Autodesk Inventor part; units mm, degrees
ref_plane "YZ Plane" through (0, 0, 0) normal (1, 0, 0) x (0, 1, 0)
ref_plane "XZ Plane" through (0, 0, 0) normal (0, 1, 0) x (-1, 0, 0)
ref_plane "XY Plane" through (0, 0, 0) normal (0, 0, 1) x (1, 0, 0)
sketch "スケッチ1" plane through (0, 0, 0) normal (0, 0, 1) x (1, 0, 0)
  line L0 (0, 0) -> (-15, 0)
  line L1 (-15, 0) -> (-15, 20)
  line L2 (-15, 20) -> (0, 20)
  line L3 (0, 20) -> (0, 0)
  line L4 (0, 0) -> (0, 43.6966) construction
  line L5 (-15, 12.5) -> (-20, 12.5)
  line L6 (-20, 12.5) -> (-20, 0)
  line L7 (-30, 0) -> (-30, 12.5)
  line L8 (-30, 0) -> (-20, 0)
  line L9 (23.8812, 0) -> (-169.724, 0) construction
  line L10 (-45, 0) -> (-45, 12.5)
  line L11 (-45, 0) -> (-35, 0)
  line L12 (-35, 12.5) -> (-35, 0)
  line L13 (-30, 12.5) -> (-35, 12.5)
  line L14 (-60, 0) -> (-60, 12.5)
  line L15 (-60, 0) -> (-50, 0)
  line L16 (-50, 12.5) -> (-50, 0)
  line L17 (-45, 12.5) -> (-50, 12.5)
  line L18 (-75, 0) -> (-75, 12.5)
  line L19 (-75, 0) -> (-65, 0)
  line L20 (-65, 12.5) -> (-65, 0)
  line L21 (-60, 12.5) -> (-65, 12.5)
  line L22 (-75, 0) -> (-80, 0)
  line L23 (-80, 0) -> (-80, 20)
  line L24 (-80, 20) -> (-75, 20)
  line L25 (-75, 20) -> (-75, 0)
  line L26 (-75, 20) -> (-15, 20)
  line L27 (-75, 0) -> (-80, 5)
  line L28 (-75, 0) -> (-67.9289, 0) construction
  line L29 (0, 5) -> (-5, 0)
  point P0 (-5, 0)
  dimension "d1" = 15
  dimension "d2" = 20
  dimension "d3" = 5
  dimension "d4" = 10
  dimension "d5" = 7.5
  dimension "d8" = 15
  dimension "d13" = 5
  dimension "d14" = 135
  dimension "d15" = 5
  dimension "d16" = 135
extrude "押し出し1" add sketch "スケッチ1" along normal blind 10 contours L0 L29 L3 | L0 L1 L2 L3 L29 | L5 L6 L8 L7 L13 L12 L11 L10 L17 L16 L15 L14 L21 L20 L19 L18 L25 L26 L1 | L25 L18 L27 L23 L24
sketch "スケッチ2" plane through (0, 0, 0) normal (0, 0, -1) x (-1, 0, 0)
  line L0 (80, 20) -> (80, 5)
  line L1 (0, 20) -> (80, 20)
  line L2 (0, 0) -> (0, 20)
  line L3 (15, 0) -> (0, 0)
  line L4 (15, 12.5) -> (15, 0)
  line L5 (20, 12.5) -> (15, 12.5)
  line L6 (20, 0) -> (20, 12.5)
  line L7 (30, 0) -> (20, 0)
  line L8 (30, 12.5) -> (30, 0)
  line L9 (35, 12.5) -> (30, 12.5)
  line L10 (35, 0) -> (35, 12.5)
  line L11 (45, 0) -> (35, 0)
  line L12 (45, 12.5) -> (45, 0)
  line L13 (50, 12.5) -> (45, 12.5)
  line L14 (50, 0) -> (50, 12.5)
  line L15 (60, 0) -> (50, 0)
  line L16 (60, 12.5) -> (60, 0)
  line L17 (65, 12.5) -> (60, 12.5)
  line L18 (65, 0) -> (65, 12.5)
  line L19 (75, 0) -> (65, 0)
  line L20 (80, 5) -> (75, 0)
  line L21 (40, 31.6917) -> (40, -9.5966) construction
  line L22 (42.5, 5) -> (37.5, 5)
  line L23 (37.5, 5) -> (37.5, 17.5)
  line L24 (37.5, 17.5) -> (42.5, 17.5)
  line L25 (42.5, 17.5) -> (42.5, 5)
  line L26 (42.5, 5) -> (37.5, 17.5) construction
  line L27 (37.5, 5) -> (42.5, 17.5) construction
  line L28 (-3.4293, 0) -> (98.1355, 0) construction
  line L29 (52.5, 5) -> (52.5, 17.5)
  line L30 (57.5, 5) -> (52.5, 5)
  line L31 (57.5, 17.5) -> (57.5, 5)
  line L32 (67.5, 5) -> (67.5, 17.5)
  line L33 (72.5, 5) -> (67.5, 5)
  line L34 (72.5, 17.5) -> (72.5, 5)
  line L35 (22.5, 5) -> (22.5, 17.5)
  line L36 (27.5, 5) -> (22.5, 5)
  line L37 (27.5, 17.5) -> (27.5, 5)
  line L38 (37.5, 5) -> (37.5, 17.5)
  line L39 (42.5, 5) -> (37.5, 5)
  line L40 (42.5, 17.5) -> (42.5, 5)
  line L41 (52.5, 5) -> (52.5, 17.5)
  line L42 (57.5, 5) -> (52.5, 5)
  line L43 (57.5, 17.5) -> (57.5, 5)
  line L44 (7.5, 5) -> (7.5, 17.5)
  line L45 (12.5, 5) -> (7.5, 5)
  line L46 (12.5, 17.5) -> (12.5, 5)
  line L47 (22.5, 5) -> (22.5, 17.5)
  line L48 (27.5, 5) -> (22.5, 5)
  line L49 (27.5, 17.5) -> (27.5, 5)
  line L50 (37.5, 5) -> (37.5, 17.5)
  line L51 (42.5, 5) -> (37.5, 5)
  line L52 (42.5, 17.5) -> (42.5, 5)
  line L53 (72.5, 17.5) -> (7.5, 17.5)
  line L54 (7.5, 15) -> (72.5, 15)
  point P0 (40, 11.25)
  point P1 (12.5, 15)
  point P2 (22.5, 15)
  point P3 (27.5, 15)
  point P4 (37.5, 15)
  point P5 (42.5, 15)
  point P6 (52.5, 15)
  point P7 (57.5, 15)
  point P8 (67.5, 15)
  dimension "d19" = 5
  dimension "d20" = 5
  dimension "d21" = 12.5
  dimension "d22" = 5
  dimension "d25" = 15
  dimension "d28" = 15
  dimension "d31" = 2.5
extrude "押し出し2" cut sketch "スケッチ2" against normal blind 7.5 contours L22 L23 L54 L25 | L54 L23 L24 L25 | L25 L53 L29 L54 | L54 L37 L53 L23 | L54 L31 L30 L29 | L29 L53 L31 L54 | L54 L35 L53 L37 | L37 L36 L35 L54 | L31 L53 L32 L54 | L54 L46 L53 L35 | L54 L34 L33 L32 | L32 L53 L34 L54 | L54 L44 L53 L46 | L46 L45 L44 L54
mirror "ミラー2" about plane through (-40, 10, 0) normal (0, 0, -1) of "押し出し1", "押し出し2"
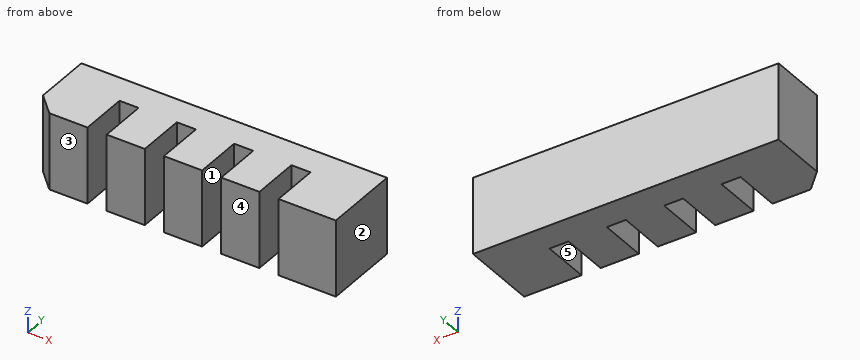
The listing builds one solid part. Answer for the finished solid, in the listing's coordinates (mm). Face numbers are marked on the shaded views. A direction names the side the tool comes from. Coordinates: 2 decimals unless noted, no trailing zeros. Write each loop counter-clockwise with the first axis right and the second up, starting at its lowest first coordinate (ties: lowest second). Pieces come first, ordered by that corner, then holes. Notation, with made-up numbers: M -28,3.5 L 31,3.5 A22 ccw 31,30.5 Z; hole C 47.25,-7.5 d5. An arc over 180 degrees is marked long. Write each question's results on one line, items separated by ' | '.
Item 1: Which of the six approach directions +Z, -Z, +X, -X, +Y, -Y give full straight-line access (tool end or side, diameter ignored) to the marked faces 4 and 5?
Answer below:
face 4: +Z, -Z, +X, -X, -Y | face 5: +Z, -Z, -Y
Item 2: The part is cut by section C-C on y = 11.25. State how many separate pieces and enclosed holes the cut face has, and give its area (3 significant figures).
Answer below:
separate pieces: 5 | enclosed holes: 5 | area: 825 mm2
Item 3: Given P1, Ø1.5, axis at x = -18.5, z = -1.5, coming from the -Y side, flat-ended and moving along its own axis, determine where the tip first touches the part or whether it passes through.
Answer below:
P1: y = 12.5
Item 4: The part is cut by section A-A on y = 1.75. Determine the outline of the cut face in (x, z), and give its area (4 significant figures).
Answer below:
outline: M -76.75,-10 L -65,-10 L -65,10 L -76.75,10 Z; M -60,-10 L -50,-10 L -50,10 L -60,10 Z; M -45,-10 L -35,-10 L -35,10 L -45,10 Z; M -30,-10 L -20,-10 L -20,10 L -30,10 Z; M -15,-10 L 0,-10 L 0,10 L -15,10 Z | area: 1,135 mm2
Item 5: Consider probe 1 along X at (y, z) = (6.5, 8.75); probe 2 along X at (y, z) = (14.5, 2.75); probe 3 along Y at (x, z) = (-65.5, 3). Determine where each line is inside the solid, lowest interval first. Write a range as [from, to].
Answer below:
probe 1: [-80, -65], [-60, -50], [-45, -35], [-30, -20], [-15, 0] | probe 2: [-80, -72.5], [-67.5, -57.5], [-52.5, -42.5], [-37.5, -27.5], [-22.5, -12.5], [-7.5, 0] | probe 3: [0, 15], [17.5, 20]
Item 6: For a pull along X with two mould halves and no side action, classify the marked faces 1, 2 and 3 as released by +X, released by -X, zero draft, split by the parting line, or undercut.
Answer below:
face 1: undercut | face 2: released by +X | face 3: zero draft
Item 7: The part is cut by section B-B on x = -16. Determine the outline of the cut face in (y, z), and give its area (4 significant figures).
Answer below:
outline: M 12.5,-10 L 20,-10 L 20,10 L 12.5,10 Z; hole M 15,-7.5 L 17.5,-7.5 L 17.5,7.5 L 15,7.5 Z | area: 112.5 mm2
